Source: CAD feature listing. Evaluate the final solid. Frame: model axes, mm. Give positions to 0.01 mm unless a question says otherwise; leave off trailing zeros. Order: outer loops, then holes, each group sorted by start corner. A loop starts at its lowest first (then second) coordinate and runs counter-clockwise, first axis right, second up.
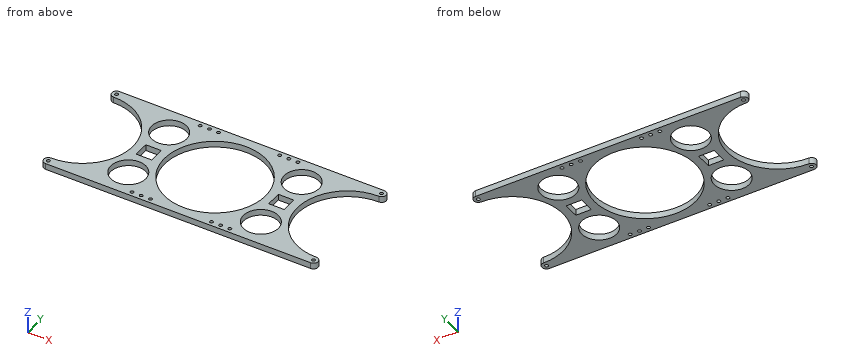
```python
from build123d import *

# Parameters (mm, degrees)
SKETCH1_R            = 82.55
SKETCH1_R_2          = 28.575
SKETCH1_W            = 25.4
SKETCH1_H            = 25.4
BOSS_EXTRUDE1_DEPTH  = 5
M5_CLEARANCE_HOLE1_D = 5.5


with BuildPart() as part:
    # Sketch1 → Boss-Extrude1 (new body, symmetric)
    with BuildSketch(Plane.XY):
        with BuildLine():
            Line((-216.868301049, 97.55), (216.868301049, 97.55))
            ThreePointArc((216.868301049, 97.55), (224.368301049, 90.05), (216.868301049, 82.55))
            ThreePointArc((216.868301049, 82.55), (134.318301049, 0), (216.868301049, -82.55))
            ThreePointArc((216.868301049, -82.55), (224.368301049, -90.05), (216.868301049, -97.55))
            Line((216.868301049, -97.55), (-216.868301049, -97.55))
            ThreePointArc((-216.868301049, -97.55), (-224.368301049, -90.05), (-216.868301049, -82.55))
            ThreePointArc((-216.868301049, -82.55), (-134.318301049, 0), (-216.868301049, 82.55))
            ThreePointArc((-216.868301049, 82.55), (-224.368301049, 90.05), (-216.868301049, 97.55))
        make_face()
        Circle(SKETCH1_R, mode=Mode.SUBTRACT)
        with Locations((108.434150525, 53.975)):
            Circle(SKETCH1_R_2, mode=Mode.SUBTRACT)
        with Locations((108.434150525, -53.975)):
            Circle(SKETCH1_R_2, mode=Mode.SUBTRACT)
        with Locations((-108.434150525, -53.975)):
            Circle(SKETCH1_R_2, mode=Mode.SUBTRACT)
        with Locations((-108.434150525, 53.975)):
            Circle(SKETCH1_R_2, mode=Mode.SUBTRACT)
        with Locations((-108.434150525, 0)):
            Rectangle(SKETCH1_W, SKETCH1_H, mode=Mode.SUBTRACT)
        with Locations((108.434150525, 0)):
            Rectangle(SKETCH1_W, SKETCH1_H, mode=Mode.SUBTRACT)
    extrude(amount=BOSS_EXTRUDE1_DEPTH, both=True)

    # M5 Clearance Hole1 (through all)
    with Locations(Plane.XY.offset(5)):
        with Locations((-80, 90.05), (-65, 90.05), (-50, 90.05), (50, 90.05), (65, 90.05), (80, 90.05), (-80, -90.05), (-65, -90.05), (-50, -90.05), (50, -90.05), (65, -90.05), (80, -90.05), (-216.868301049, 90.05), (216.868301049, 90.05), (-216.868301049, -90.05), (216.868301049, -90.05)):
            Hole(M5_CLEARANCE_HOLE1_D / 2)


solid = part.part
```
1) Pin query (flat end, axial travel): pin 1 (3 mm diameter, centred on y = -4.5, z = 0, fed in from +X); pin 2 (2 mm diameter, centred on y = -48, z = -0.5, fed in from +X); pin 3 (5 mm diameter, centred on y = -53.5, z = 2, fed in from -X). Return the tip coordinate at first contact, or that it passes through.
Report:
pin 1: stops at x = 134.54
pin 2: stops at x = 150.43
pin 3: stops at x = -156.22
2) Section query B-B, the plane y = -74.5. Return the cut outline in (x, z), and give its area (3 significant figures).
Report:
outline: (-181.31, -5) - (-128.32, -5) - (-128.32, 5) - (-181.31, 5) - close; (-88.55, -5) - (-35.56, -5) - (-35.56, 5) - (-88.55, 5) - close; (35.56, -5) - (88.55, -5) - (88.55, 5) - (35.56, 5) - close; (128.32, -5) - (181.31, -5) - (181.31, 5) - (128.32, 5) - close
area: 2,120 mm2
3) Section query C-C, the plane x = 108. Return the cut outline in (y, z), and give its area (3 significant figures).
Report:
outline: (-97.55, -5) - (-82.55, -5) - (-82.55, 5) - (-97.55, 5) - close; (-25.4, -5) - (-12.7, -5) - (-12.7, 5) - (-25.4, 5) - close; (12.7, -5) - (25.4, -5) - (25.4, 5) - (12.7, 5) - close; (82.55, -5) - (97.55, -5) - (97.55, 5) - (82.55, 5) - close
area: 554 mm2
4) Material intervals for L1, parallel to Y at x = 108, z = -3.5; L2, parallel to Y at x = 50, z = 2.25; L3, parallel to Y at x = 0, z = 2.75, sorted ascending.
Report:
L1: y = -97.55 to -82.55, -25.4 to -12.7, 12.7 to 25.4, 82.55 to 97.55
L2: y = -97.55 to -92.8, -87.3 to -65.68, 65.68 to 87.3, 92.8 to 97.55
L3: y = -97.55 to -82.55, 82.55 to 97.55
5) Section query A-A, the plane x = 0. Return the cut outline in (y, z), and give its area (3 significant figures).
Report:
outline: (-97.55, -5) - (-82.55, -5) - (-82.55, 5) - (-97.55, 5) - close; (82.55, -5) - (97.55, -5) - (97.55, 5) - (82.55, 5) - close
area: 300 mm2
6) Section query D-D, the plane z = -1.75. Count the separate pieces of the cut face and the enclosed holes in it, and give its area (3 significant figures).
Report:
separate pieces: 1
enclosed holes: 23
area: 30,200 mm2
